from build123d import *
from OCP.BRepFilletAPI import BRepFilletAPI_MakeChamfer

# Parameters (mm, degrees)
BOSS_EXTRUDE1_DEPTH = 6
SKETCH2_R           = 2.25
CUT_EXTRUDE1_DEPTH  = 29.948229652
CHAMFER1_SIZE       = 2
CHAMFER1_SIZE2      = 3.464101615
CHAMFER3_SIZE       = 1
CHAMFER4_SIZE       = 1
FILLET1_R           = 5


with BuildPart() as part:
    # Sketch1 → Boss-Extrude1 (new, symmetric)
    with BuildSketch(Plane(origin=(0, 0, 0), x_dir=(0, 0, -1), z_dir=(1, 0, 0))):
        Polygon((7.5, 6), (11.5, 6), (11.5, -11), (12.1, -11), (12.1, -19), (11.5, -19), (11.5, -21), (7.5, -21), (7.5, -4), (-11.5, -4), (-11.5, 6), (-7.5, 6), (-7.5, 0), (7.5, 0), align=None)
    extrude(amount=BOSS_EXTRUDE1_DEPTH, both=True)

    # Sketch2 → Cut-Extrude1 (cut, through all)
    with BuildSketch(Plane.XY.offset(-7.5)):
        with Locations((0, -15)):
            Circle(SKETCH2_R)
    extrude(amount=-CUT_EXTRUDE1_DEPTH, mode=Mode.SUBTRACT)

    # Chamfer1: one chamfer whose edges measure the first distance from different faces: ONE call of the kernel's chamfer builder (chamfer() names one face for all edges)
    chamfer1_edges_1 = [part.edges().sort_by_distance(p)[0] for p in [
        (0, 6, -7.5),
    ]]
    chamfer1_side_1 = [part.faces().sort_by_distance(p)[0] for p in [
        (0, 6, -9.5),
    ]]
    chamfer1_edges_2 = [part.edges().sort_by_distance(p)[0] for p in [
        (0, 6, 7.5),
    ]]
    chamfer1_side_2 = [part.faces().sort_by_distance(p)[0] for p in [
        (0, 6, 9.5),
    ]]
    chamfer1 = BRepFilletAPI_MakeChamfer(part.part.solid().wrapped)
    for e in chamfer1_edges_1:
        chamfer1.Add(CHAMFER1_SIZE, CHAMFER1_SIZE2, e.wrapped, chamfer1_side_1[0].wrapped)  # the first distance lies on this face
    for e in chamfer1_edges_2:
        chamfer1.Add(CHAMFER1_SIZE, CHAMFER1_SIZE2, e.wrapped, chamfer1_side_2[0].wrapped)  # the first distance lies on this face
    add(Compound.cast(chamfer1.Shape()), mode=Mode.REPLACE)

    # Chamfer3
    chamfer3_edges = [part.edges().sort_by_distance(p)[0] for p in [
        (-6, 4.267949192, -8.5),
        (-6, 4.267949192, 8.5),
        (6, 4.267949192, -8.5),
        (6, 4.267949192, 8.5),
    ]]
    chamfer(chamfer3_edges, length=CHAMFER3_SIZE)

    # Chamfer4
    chamfer4_edges = [part.edges().sort_by_distance(p)[0] for p in [
        (-6, -21, -9.5),
        (6, -21, -9.5),
    ]]
    chamfer(chamfer4_edges, length=CHAMFER4_SIZE)

    # Fillet1
    fillet1_edges = [part.edges().sort_by_distance(p)[0] for p in [
        (0, -4, -7.5),
    ]]
    fillet(fillet1_edges, radius=FILLET1_R)


solid = part.part
Could you check a few things on this model? Use its own coordinates, in mm. A direction names the side the tool comes from. Round coordinates to 2 decimals unless told otherwise and drop trailing zeros. Write each loop counter-clockwise with the first axis right and the second up, starting at its lowest first coordinate (ties: lowest second). Pieces come first, ordered by that corner, then holes. Notation, with made-up numbers: (9.5, 68) - (35.5, 68) arc R20 ccw to (35.5, 86) - close; hole circle Ø2 at (8.25, -7). An arc over 180 degrees is marked (long way). Use a Markdown table: item, result.
Q1. I want a section at C-C (x = 4.25). List the corners of the cut face in (y, z) for me, plus the area to 3 significant figures.
Output values:
| item | result |
|---|---|
| outline | (-21, -11.5) - (-19, -11.5) - (-19, -12.1) - (-11, -12.1) - (-11, -11.5) - (6, -11.5) - (6, -9.5) - (2.54, -7.5) - (0, -7.5) - (0, 7.5) - (2.54, 7.5) - (6, 9.5) - (6, 11.5) - (-4, 11.5) - (-4, -2.5) arc R5 cw to (-9, -7.5) - (-21, -7.5) - close |
| area | 211 mm2 |
Q2. Thinking about a two-plate mould opening in Z: for faces 4 (the flat face through (0, -20, -11.5)), 5 (the flat face through (-5.5, -20.5, -9.5)), 6 (the flat face through (-5.49, 3.56, 8.66)), which applies, released by +Z, released by -Z, zero draft, split by the parting line, or undercut?
Output values:
| item | result |
|---|---|
| face 4 | released by -Z |
| face 5 | zero draft |
| face 6 | undercut |
Q3. I want a section at A-A (y = -15). List the corners of the cut face in (x, z) for me.
Output values:
| item | result |
|---|---|
| outline | (-6, -12.1) - (-2.25, -12.1) - (-2.25, -7.5) - (-6, -7.5) - close; (2.25, -12.1) - (6, -12.1) - (6, -7.5) - (2.25, -7.5) - close |
Q4. Please list where these lines run through material, in increasing order: L1, parallel to Y at x = 0, z = -11; L2, parallel to Z at x = -4.5, y = 0.75; L3, parallel to Y at x = 1, z = 1.5.
Output values:
| item | result |
|---|---|
| L1 | -21 to -17.25, -12.75 to 6 |
| L2 | -11.5 to -7.5, 7.5 to 11.5 |
| L3 | -4 to 0 |
Q5. For pin 1 (2 mm diameter, centred on x = 3, y = -0.5, fed in from -Z); pin 2 (5 mm diameter, centred on x = 0, z = 2, fed in from -Y), each with a flat end and sliding along its axis, tell me the tip position at first contact or that it passes through.
Output values:
| item | result |
|---|---|
| pin 1 | z = -11.5 |
| pin 2 | y = -4 |
Q6. I want a section at D-D (y = -6). List the corners of the cut face in (x, z) for me, plus the area to 3 significant figures.
Output values:
| item | result |
|---|---|
| outline | (-6, -11.5) - (6, -11.5) - (6, -6.5) - (-6, -6.5) - close |
| area | 60.0 mm2 |
Q7. I want a section at B-B (x = 0). List the corners of the cut face in (y, z) for me.
Output values:
| item | result |
|---|---|
| outline | (-21, -11.5) - (-19, -11.5) - (-19, -12.1) - (-17.25, -12.1) - (-17.25, -7.5) - (-21, -7.5) - close; (-12.75, -12.1) - (-11, -12.1) - (-11, -11.5) - (6, -11.5) - (6, -9.5) - (2.54, -7.5) - (0, -7.5) - (0, 7.5) - (2.54, 7.5) - (6, 9.5) - (6, 11.5) - (-4, 11.5) - (-4, -2.5) arc R5 cw to (-9, -7.5) - (-12.75, -7.5) - close |
Q8. For faces 1 (the flat face through (0, -4, 4)), 2 (the flat face through (0, 0, 0)), 3 (the flat face through (5.49, 3.56, 8.66)), which set-ups out of +Z, -Z, +X, -X, +Y, -Y let a thin tool reach every point of the face, with its end or its side?
Output values:
| item | result |
|---|---|
| face 1 | +Z, +X, -X, -Y |
| face 2 | +X, -X, +Y |
| face 3 | +X, +Y |
